from build123d import *

# Parameters (mm, degrees)
ESQUISSE2_R                   = 3
ESQUISSE2_R_2                 = 10.1
ESQUISSE2_R_3                 = 1.5
ESQUISSE2_R_4                 = 4.1
ESQUISSE2_W                   = 25
ESQUISSE2_H                   = 60
ESQUISSE2_W_2                 = 20
ESQUISSE2_H_2                 = 30
BOSS_EXTRU_1_DEPTH            = 5
CONG_2_R                      = 2
DIAM_TRE_DU_PER_AGE_3_0_3_1_D = 3
ESQUISSE6_R                   = 1.495854397
ESQUISSE6_R_2                 = 1.51008819
ENL_V_MAT_EXTRU_1_DEPTH       = 10


with BuildPart() as part:
    # Esquisse2 → Boss.-Extru.1 (new body)
    with BuildSketch(Plane(origin=(0, 0, 0), x_dir=(1, 0, 0), z_dir=(0, 1, 0))):
        Polygon((-140, 95), (-140, -95), (-116, -105), (-87, -105), (-87, -40), (-45, -40), (-45, -25), (45, -25), (45, -40), (87, -40), (87, -105), (116, -105), (140, -95), (140, 95), (116, 105), (87, 105), (87, 40), (45, 40), (45, 25), (-45, 25), (-45, 40), (-87, 40), (-87, 105), (-116, 105), align=None)
        with Locations(Location((-96, 30, 0), (0, 0, 270))):
            Circle(ESQUISSE2_R, mode=Mode.SUBTRACT)
        with Locations(Location((-96, -30, 0), (0, 0, 270))):
            Circle(ESQUISSE2_R, mode=Mode.SUBTRACT)
        with Locations(Location((-55, -30, 0), (0, 0, 270))):
            Circle(ESQUISSE2_R, mode=Mode.SUBTRACT)
        with Locations(Location((-55, 30, 0), (0, 0, 270))):
            Circle(ESQUISSE2_R, mode=Mode.SUBTRACT)
        with Locations(Location((-130, 85, 0), (0, 0, 270))):
            Circle(ESQUISSE2_R, mode=Mode.SUBTRACT)
        with Locations(Location((-130, -85, 0), (0, 0, 270))):
            Circle(ESQUISSE2_R, mode=Mode.SUBTRACT)
        with Locations(Location((-102.7, 89.3, 0), (0, 0, 270))):
            Circle(ESQUISSE2_R_2, mode=Mode.SUBTRACT)
        with Locations(Location((-90, 89.3, 0), (0, 0, 270))):
            Circle(ESQUISSE2_R_3, mode=Mode.SUBTRACT)
        with Locations(Location((-102.7, 102, 0), (0, 0, 270))):
            Circle(ESQUISSE2_R_3, mode=Mode.SUBTRACT)
        with Locations(Location((-115.4, 89.3, 0), (0, 0, 270))):
            Circle(ESQUISSE2_R_3, mode=Mode.SUBTRACT)
        with Locations(Location((-102.7, 76.6, 0), (0, 0, 270))):
            Circle(ESQUISSE2_R_3, mode=Mode.SUBTRACT)
        with Locations(Location((-102.7, -89.3, 0), (0, 0, 270))):
            Circle(ESQUISSE2_R_2, mode=Mode.SUBTRACT)
        with Locations(Location((-90, -89.3, 0), (0, 0, 270))):
            Circle(ESQUISSE2_R_3, mode=Mode.SUBTRACT)
        with Locations(Location((-102.7, -76.6, 0), (0, 0, 270))):
            Circle(ESQUISSE2_R_3, mode=Mode.SUBTRACT)
        with Locations(Location((-115.4, -89.3, 0), (0, 0, 270))):
            Circle(ESQUISSE2_R_3, mode=Mode.SUBTRACT)
        with Locations(Location((-102.7, -102, 0), (0, 0, 270))):
            Circle(ESQUISSE2_R_3, mode=Mode.SUBTRACT)
        with Locations(Location((102.7, -102, 0), (0, 0, 90))):
            Circle(ESQUISSE2_R_3, mode=Mode.SUBTRACT)
        with Locations(Location((115.4, -89.3, 0), (0, 0, 90))):
            Circle(ESQUISSE2_R_3, mode=Mode.SUBTRACT)
        with Locations(Location((102.7, -76.6, 0), (0, 0, 90))):
            Circle(ESQUISSE2_R_3, mode=Mode.SUBTRACT)
        with Locations(Location((90, -89.3, 0), (0, 0, 90))):
            Circle(ESQUISSE2_R_3, mode=Mode.SUBTRACT)
        with Locations(Location((102.7, -89.3, 0), (0, 0, 90))):
            Circle(ESQUISSE2_R_2, mode=Mode.SUBTRACT)
        with Locations(Location((102.7, 76.6, 0), (0, 0, 90))):
            Circle(ESQUISSE2_R_3, mode=Mode.SUBTRACT)
        with Locations(Location((115.4, 89.3, 0), (0, 0, 90))):
            Circle(ESQUISSE2_R_3, mode=Mode.SUBTRACT)
        with Locations(Location((102.7, 102, 0), (0, 0, 90))):
            Circle(ESQUISSE2_R_3, mode=Mode.SUBTRACT)
        with Locations(Location((90, 89.3, 0), (0, 0, 90))):
            Circle(ESQUISSE2_R_3, mode=Mode.SUBTRACT)
        with Locations(Location((102.7, 89.3, 0), (0, 0, 90))):
            Circle(ESQUISSE2_R_2, mode=Mode.SUBTRACT)
        with Locations(Location((130, -85, 0), (0, 0, 90))):
            Circle(ESQUISSE2_R, mode=Mode.SUBTRACT)
        with Locations(Location((130, 85, 0), (0, 0, 90))):
            Circle(ESQUISSE2_R, mode=Mode.SUBTRACT)
        with Locations(Location((55, 30, 0), (0, 0, 90))):
            Circle(ESQUISSE2_R, mode=Mode.SUBTRACT)
        with Locations(Location((55, -30, 0), (0, 0, 90))):
            Circle(ESQUISSE2_R, mode=Mode.SUBTRACT)
        with Locations(Location((96, -30, 0), (0, 0, 90))):
            Circle(ESQUISSE2_R, mode=Mode.SUBTRACT)
        with Locations(Location((96, 30, 0), (0, 0, 90))):
            Circle(ESQUISSE2_R, mode=Mode.SUBTRACT)
        with Locations(Location((-129, 40.5, 0), (0, 0, 270))):
            Circle(ESQUISSE2_R_4, mode=Mode.SUBTRACT)
        with Locations(Location((-129, -40.5, 0), (0, 0, 270))):
            Circle(ESQUISSE2_R_4, mode=Mode.SUBTRACT)
        with Locations(Location((129, -40.5, 0), (0, 0, 90))):
            Circle(ESQUISSE2_R_4, mode=Mode.SUBTRACT)
        with Locations(Location((129, 40.5, 0), (0, 0, 90))):
            Circle(ESQUISSE2_R_4, mode=Mode.SUBTRACT)
        with Locations(Location((0, 0, 0), (0, 0, 270))):
            Circle(ESQUISSE2_R, mode=Mode.SUBTRACT)
        with Locations((-72.5, 0)):
            Rectangle(ESQUISSE2_W, ESQUISSE2_H, mode=Mode.SUBTRACT)
        with BuildLine():
            Line((-123, 22), (-123, -22))
            ThreePointArc((-123, -22), (-128, -27), (-133, -22))
            Line((-133, -22), (-133, 22))
            ThreePointArc((-133, 22), (-128, 27), (-123, 22))
        make_face(mode=Mode.SUBTRACT)
        with Locations((-109, 0)):
            Rectangle(ESQUISSE2_W_2, ESQUISSE2_H_2, mode=Mode.SUBTRACT)
        with Locations((109, 0)):
            Rectangle(ESQUISSE2_W_2, ESQUISSE2_H_2, mode=Mode.SUBTRACT)
        with Locations((72.5, 0)):
            Rectangle(ESQUISSE2_W, ESQUISSE2_H, mode=Mode.SUBTRACT)
        with BuildLine():
            Line((123, 22), (123, -22))
            ThreePointArc((123, -22), (128, -27), (133, -22))
            Line((133, -22), (133, 22))
            ThreePointArc((133, 22), (128, 27), (123, 22))
        make_face(mode=Mode.SUBTRACT)
    extrude(amount=BOSS_EXTRU_1_DEPTH)

    # Congé2
    cong_2_edges = [part.edges().sort_by_distance(p)[0] for p in [
        (-87, 2.5, -105),
        (-45, 2.5, -40),
        (45, 2.5, -40),
        (87, 2.5, -105),
        (87, 2.5, 105),
        (45, 2.5, 40),
        (-45, 2.5, 40),
        (-87, 2.5, 105),
    ]]
    fillet(cong_2_edges, radius=CONG_2_R)

    # Diamètre du perçage Ø3.0 (3)1 (through all)
    with Locations(Plane(origin=(0, 5, 0), x_dir=(1, 0, 0), z_dir=(0, 1, 0))):
        with Locations((-92, 69.3), (-92, 49.3), (-20, 20), (0, 20), (20, 20), (20, -20), (0, -20), (-20, -20), (-92, -69.3), (-92, -49.3), (92, -69.3), (92, -49.3), (92, 69.3), (92, 49.3), (112, 69.3), (112, 49.3), (-112, 69.3), (-112, 49.3), (-112, -49.3), (-112, -69.3), (112, -69.3), (112, -49.3), (40, -20), (40, 20), (-40, 20), (-40, -20)):
            Hole(DIAM_TRE_DU_PER_AGE_3_0_3_1_D / 2)

    # Esquisse6 → Enlèv. mat.-Extru.1 (cut)
    with BuildSketch(Plane.XZ):
        with Locations((112.218706977, 95.273590322)):
            Circle(ESQUISSE6_R)
        with Locations(Location((91.995720379, 95.273590322, 0), (0, 0, 270))):
            Circle(ESQUISSE6_R_2)
    extrude(amount=-ENL_V_MAT_EXTRU_1_DEPTH, mode=Mode.SUBTRACT)


solid = part.part
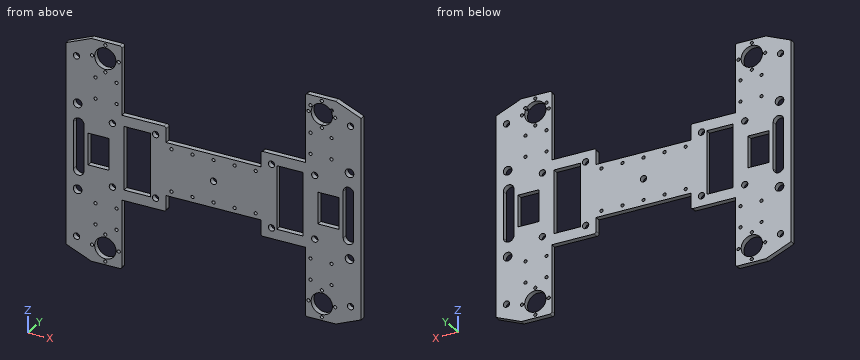
Build history of the part. All positions in model axes, mm. Round coordinates to 2 decimals unless told otherwise and drop trailing zeros. Write each loop counter-clockwise with the first axis right and the second up, starting at its lowest first coordinate (ties: lowest second). Pieces come first, ordered by that corner, then holes. Notation, with made-up numbers: (79, -26.5) - (122, -26.5) arc R34 ccw to (122, 12.5) - close; hole circle Ø5 at (-26, 80.5). An arc over 180 degrees is marked (long way). Use CSV: the item, a comma, the result in double quotes.
(1) Band-saw the part on A-A (z = 0). Give the number of separate pieces and of enclosed holes in the cut face, plus the area to 3 significant figures.
Response:
separate pieces,"8"
enclosed holes,"0"
area,"820 mm²"
(2) Wall check: line 1 (X direction, y = 2.1, z = 76.6); line 2 (Z direction, x = -92, y = 4.25); line 3 (X direction, y = 2.65, z = 49.3). Give the ranges that are in metal, low to high.
Response:
line 1,"-140 to -104.2, -101.2 to -87, 87 to 101.2, 104.2 to 140"
line 2,"-105 to -70.8, -67.8 to -50.8, -47.8 to 47.8, 50.8 to 67.8, 70.8 to 105"
line 3,"-140 to -113.5, -110.5 to -93.5, -90.5 to -87, 87 to 90.5, 93.5 to 110.5, 113.5 to 140"
(3) Band-saw the part on B-B (z = 62). Write the cut outline in (x, y), plus the area to 3 significant figures.
Response:
outline,"(-140, 0) - (-87, 0) - (-87, 5) - (-140, 5) - close; (87, 0) - (140, 0) - (140, 5) - (87, 5) - close"
area,"530 mm²"
